Geometry check sheet. Reference: drawing and pictorial views, mm from the part's lowest x, y, z. A direction names the side the tool comes from. Round coordinates to 2 decimals unless told otherwise and drop trailing zeros. Write each loop counter-clockwise with the first axis right and the second up, starting at its lowest first coordinate (ties: lowest second). Pieces come first, ordered by that corner, then holes. Notation, with made-up numbers: M 61.25,18 L 110.25,18 A13 ccw 110.25,39 Z; hole C -37,60.25 d6. An arc over 180 degrees is marked long. Answer in a Markdown table with one row per item. Add a question column.
1. Go/stop test with flat-tipped pins: pin 1 Ø2.5 at (x, y) = (20.5, 37) entering from -Z (3 decimals); pin 2 Ø8 at (x, y) = (21.5, 20) entering from +Z (3 decimals); pin 3 Ø6.5 at (x, y) = (93.853, 11.43) entering from +Z (3 decimals). Record where each tip stops, or that it passes through.
2. Material ranges on probe 1 along Y at (x, z) = (56, 37); probe 2 along X at (y, z) = (24.5, 15); probe 3 along X at (y, z) = (11, 2), recorded low to high.
3. Sectioned sample at B-B on y = 11.43. Record the cut outline in (x, z) (3 decimals).
4. Sectioned sample at D-D on x = 72.5. Record the cut outline in (y, z) (3 decimals), plus the area to 3 significant figures.
5. Draft check along Y on the marked faces 1, 2 and 3. Enter one of: pulls with the +Y half, pulls with the -Y half, needs draft (parallel to the pull), parting line crosses it, or undercut.
6. Sectioned sample at C-C on z = 43.5. Record the cut outline in (x, y), plus the area to 3 significant figures.
7. Sectioned sample at A-A on x = 11.43. Record the cut outline in (y, z) (3 decimals).
8. Set-up check for the marked faces 4 and 5: record each of +Z, -Z, +X, -X, +Y, -Y from which the full face is reachable in a straight line by a thin tool's end or side.
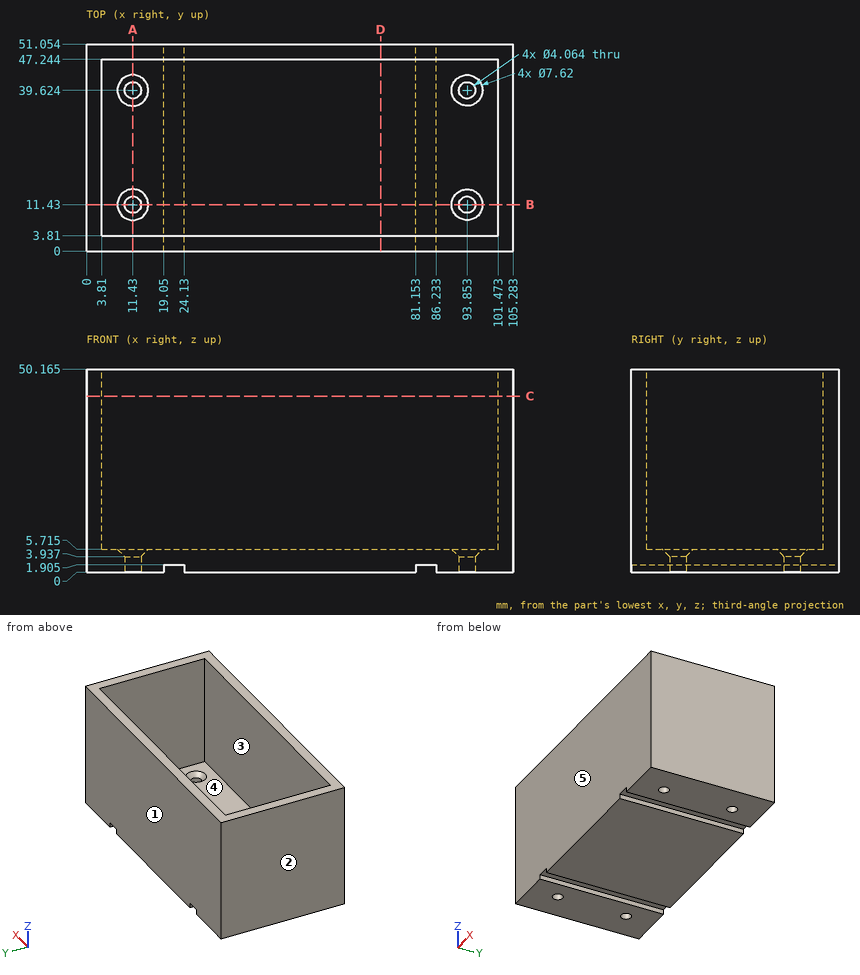
Geometry check:
| question | item | result |
|---|---|---|
| 1 | pin 1 | stops at z = 1.905 |
| 1 | pin 2 | stops at z = 5.715 |
| 1 | pin 3 | stops at z = 5.155 |
| 2 | probe 1 | y = 0 to 3.81, 47.24 to 51.05 |
| 2 | probe 2 | x = 0 to 3.81, 101.47 to 105.28 |
| 2 | probe 3 | x = 0 to 9.44, 13.42 to 91.87, 95.84 to 105.28 |
| 3 | outline | M 0,0 L 9.398,0 L 9.398,3.937 L 7.62,5.715 L 3.81,5.715 L 3.81,50.165 L 0,50.165 Z; M 13.462,0 L 19.05,0 L 19.05,1.905 L 24.13,1.905 L 24.13,0 L 81.153,0 L 81.153,1.905 L 86.233,1.905 L 86.233,0 L 91.821,0 L 91.821,3.937 L 90.043,5.715 L 15.24,5.715 L 13.462,3.937 Z; M 95.885,0 L 105.283,0 L 105.283,50.165 L 101.473,50.165 L 101.473,5.715 L 97.663,5.715 L 95.885,3.937 Z |
| 4 | outline | M 0,0 L 51.054,0 L 51.054,50.165 L 47.244,50.165 L 47.244,5.715 L 3.81,5.715 L 3.81,50.165 L 0,50.165 Z |
| 4 | area | 630 mm2 |
| 5 | face 1 | pulls with the +Y half |
| 5 | face 2 | needs draft |
| 5 | face 3 | undercut |
| 6 | outline | M 0,0 L 105.28,0 L 105.28,51.05 L 0,51.05 Z; hole M 3.81,3.81 L 101.47,3.81 L 101.47,47.24 L 3.81,47.24 Z |
| 6 | area | 1,130 mm2 |
| 7 | outline | M 0,0 L 9.398,0 L 9.398,3.937 L 7.62,5.715 L 3.81,5.715 L 3.81,50.165 L 0,50.165 Z; M 13.462,0 L 37.592,0 L 37.592,3.937 L 35.814,5.715 L 15.24,5.715 L 13.462,3.937 Z; M 41.656,0 L 51.054,0 L 51.054,50.165 L 47.244,50.165 L 47.244,5.715 L 43.434,5.715 L 41.656,3.937 Z |
| 8 | face 4 | +Z |
| 8 | face 5 | +Z, -Z, +X, -X, -Y |
